Could you check a few things on this model? Use its own coordinates, in mm. Give positions to 0.01 mm unless a question says otherwise; leave off trailing zeros. Write each loop counter-clockwise with the first axis right and the second up, starting at its lowest first coordinate (ties: lowest second). Pieces come first, ordered by that corner, then holes. Notation, with made-up numbers: M -40,76 L -30,76 A13 ccw -30,92 Z; hole C -14,77 d5. An arc over 180 degrees is marked long. Answer as CSV lines item,"result". Start each with the question number.
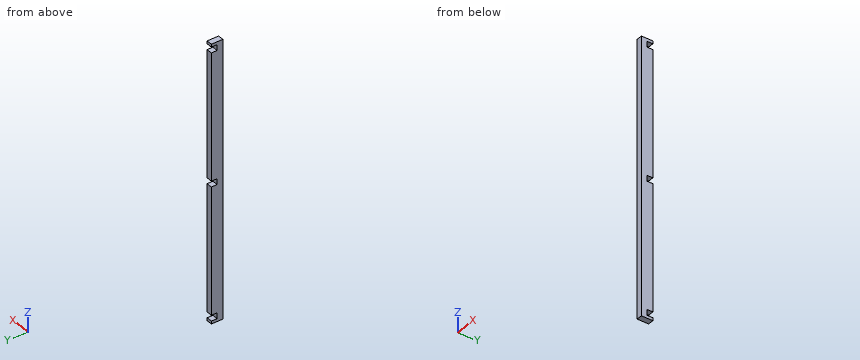
from build123d import *

# Parameters (mm, degrees)
SKETCH1_W               = 50.8
SKETCH1_H               = 101.6
BOSS_EXTRUDE1_DEPTH     = 2438.4
CUT_EXTRUDE1_DEPTH      = 2440.45810376
CUT_EXTRUDE1_DEPTH_BACK = 2440.45810376
SKETCH2_W               = 50.8
SKETCH2_H               = 50.8


with BuildPart() as part:
    # Sketch1 → Boss-Extrude1 (new body)
    with BuildSketch(Plane.XY):
        Rectangle(SKETCH1_W, SKETCH1_H)
    extrude(amount=BOSS_EXTRUDE1_DEPTH)

    # Sketch2 → Cut-Extrude1 (cut, two sides: drawn at the far end of the back side and taken through both)
    with BuildSketch(Plane(origin=(25.4, 0, 0), x_dir=(0, 0, -1), z_dir=(1, 0, 0)).offset(-CUT_EXTRUDE1_DEPTH_BACK)):
        with Locations((-1219.2, 25.4)):
            Rectangle(SKETCH2_W, SKETCH2_H)
        with Locations((-2387.6, 25.4)):
            Rectangle(SKETCH2_W, SKETCH2_H)
        with Locations((-50.8, 25.4)):
            Rectangle(SKETCH2_W, SKETCH2_H)
    extrude(amount=CUT_EXTRUDE1_DEPTH + CUT_EXTRUDE1_DEPTH_BACK, mode=Mode.SUBTRACT)


solid = part.part
1. Imagine slicing it at A-A, the plane x = 3. Please give me the cut outline in (y, z), plus the area to 3 significant figures.
2. Will this pin go through, and if not, where does the flat tip stop? P1, Ø1.5, axis at x = -16, z = 1195, coming from the +Y side.
3. Please list where these lines run through material, in increasing order: line 1 (Z direction, x = -11.5, y = 15); line 2 (Y direction, x = -9.5, z = 1240.5).
Solutions:
1,outline,"M -50.8,0 L 50.8,0 L 50.8,25.4 L 0,25.4 L 0,76.2 L 50.8,76.2 L 50.8,1193.8 L 0,1193.8 L 0,1244.6 L 50.8,1244.6 L 50.8,2362.2 L 0,2362.2 L 0,2413 L 50.8,2413 L 50.8,2438.4 L -50.8,2438.4 Z"
1,area,"240,000 mm²"
2,P1,"y = 0"
3,line 1,"0 to 25.4, 76.2 to 1193.8, 1244.6 to 2362.2, 2413 to 2438.4"
3,line 2,"-50.8 to 0"
